from build123d import *

# Parameters (mm, degrees)
F0_W     = 64
F0_H     = 16
F1_DEPTH = 9
F2_R     = 2.5
F3_DEPTH = 2
F4_W     = 61
F4_H     = 13
F4_R     = 3.25
F4_R_2   = 2.5
F5_DEPTH = 8
F6_R     = 1.25
F7_DEPTH = 10


with BuildPart() as f1:
    # F0 (on Top) → F1 (new body)
    with BuildSketch(Plane.XY):
        Rectangle(F0_W, F0_H)
    extrude(amount=F1_DEPTH)

    # F2 (on face) → F3 (join)
    with BuildSketch(Plane.XY.offset(9)):
        with Locations((-28, 4)):
            Circle(F2_R)
        with Locations((-28, -4)):
            Circle(F2_R)
        with Locations((-20, 4)):
            Circle(F2_R)
        with Locations((-20, -4)):
            Circle(F2_R)
        with Locations((-12, 4)):
            Circle(F2_R)
        with Locations((-12, -4)):
            Circle(F2_R)
        with Locations((-4, 4)):
            Circle(F2_R)
        with Locations((-4, -4)):
            Circle(F2_R)
        with Locations((4, 4)):
            Circle(F2_R)
        with Locations((4, -4)):
            Circle(F2_R)
        with Locations((12, 4)):
            Circle(F2_R)
        with Locations((12, -4)):
            Circle(F2_R)
        with Locations((20, 4)):
            Circle(F2_R)
        with Locations((20, -4)):
            Circle(F2_R)
        with Locations((28, 4)):
            Circle(F2_R)
        with Locations((28, -4)):
            Circle(F2_R)
    extrude(amount=F3_DEPTH)

    # F4 (on face) → F5 (cut)
    with BuildSketch(Plane(origin=(0, 0, 0), x_dir=(1, 0, 0), z_dir=(0, 0, -1))):
        Rectangle(F4_W, F4_H)
        with Locations((-24, 0)):
            Circle(F4_R, mode=Mode.SUBTRACT)
        with Locations((-16, 0)):
            Circle(F4_R, mode=Mode.SUBTRACT)
        with Locations((-8, 0)):
            Circle(F4_R, mode=Mode.SUBTRACT)
        Circle(F4_R, mode=Mode.SUBTRACT)
        with Locations((8, 0)):
            Circle(F4_R, mode=Mode.SUBTRACT)
        with Locations((16, 0)):
            Circle(F4_R, mode=Mode.SUBTRACT)
        with Locations((24, 0)):
            Circle(F4_R, mode=Mode.SUBTRACT)
        with Locations((-24, 0)):
            Circle(F4_R_2)
        with Locations((-16, 0)):
            Circle(F4_R_2)
        with Locations((-8, 0)):
            Circle(F4_R_2)
        Circle(F4_R_2)
        with Locations((8, 0)):
            Circle(F4_R_2)
        with Locations((16, 0)):
            Circle(F4_R_2)
        with Locations((24, 0)):
            Circle(F4_R_2)
    extrude(amount=-F5_DEPTH, mode=Mode.SUBTRACT)

    # F6 (on face) → F7 (cut)
    with BuildSketch(Plane(origin=(0, 0, 0), x_dir=(1, 0, 0), z_dir=(0, 0, -1))):
        with Locations((-28, 4)):
            Circle(F6_R)
        with Locations((-28, -4)):
            Circle(F6_R)
        with Locations((-20, 4)):
            Circle(F6_R)
        with Locations((-20, -4)):
            Circle(F6_R)
        with Locations((-12, 4)):
            Circle(F6_R)
        with Locations((-12, -4)):
            Circle(F6_R)
        with Locations((-4, 4)):
            Circle(F6_R)
        with Locations((-4, -4)):
            Circle(F6_R)
        with Locations((4, 4)):
            Circle(F6_R)
        with Locations((4, -4)):
            Circle(F6_R)
        with Locations((12, 4)):
            Circle(F6_R)
        with Locations((12, -4)):
            Circle(F6_R)
        with Locations((20, 4)):
            Circle(F6_R)
        with Locations((20, -4)):
            Circle(F6_R)
        with Locations((28, 4)):
            Circle(F6_R)
        with Locations((28, -4)):
            Circle(F6_R)
    extrude(amount=-F7_DEPTH, mode=Mode.SUBTRACT)


solid = f1.part
Verification items for the finished model (mm, model axes). A direction names the side the tool comes from. Round coordinates to 2 decimals unless told otherwise and drop trailing zeros. Loops run counter-clockwise (first coordinate to the right, second up) from the corner with the lowest first, then second, coordinate; pieces in that order, holes last. Notation, with made-up numbers: (-33.75, 11) - (-6.75, 11) arc R31 ccw to (-6.75, 48) - close; hole circle Ø2 at (-16.5, 62). An arc over 180 degrees is marked (long way). Write item = value, one per line.
Q1. Sectioned sample at A-A on z = 4.5. State how many separate pieces and enclosed holes the cut face has, plus the area to 3 significant figures.
Here are the results:
separate_pieces = 8
enclosed_holes = 8
area = 326 mm^2
Q2. Tool access check on faces 1 (the cylindrical face through (4.577, 5.109, 8.986)), 2 (the flat face through (-12, 4, 11)), 3 (the cylindrical face through (-14.5, 4.1, 10)). Record the directions out of +Z, -Z, +X, -X, +Y, -Y that give a thin tool (end or side, any length) a straight path to the whole face; none if there is none.
Here are the results:
face_1 = -Z
face_2 = +Z, +X, -X, +Y, -Y
face_3 = +Z
Q3. Sectioned sample at B-B on x = -16. Record the boundary of the cut face in (y, z).
Here are the results:
outline = (-8, 0) - (-6.5, 0) - (-6.5, 8) - (-3.25, 8) - (-3.25, 0) - (-2.5, 0) - (-2.5, 8) - (2.5, 8) - (2.5, 0) - (3.25, 0) - (3.25, 8) - (6.5, 8) - (6.5, 0) - (8, 0) - (8, 9) - (-8, 9) - close
Q4. Depth check by flat-ended pin: pin 1 (2 mm diameter, centred on x = -28, y = 4, fed in from -Z); pin 2 (3 mm diameter, centred on x = 4, y = -4, fed in from -Z); pin 3 (6 mm diameter, centred on x = 24, y = 0, fed in from +Z). Enter the tip coordinate at first touch or a pass-through.
Here are the results:
pin_1 = 10
pin_2 = 8
pin_3 = 9
Q5. Material ranges on L1, parallel to Y at x = -12, z = 8.5; L2, parallel to Y at x = -16, z = 4; L3, parallel to Y at x = -20, z = 9.25, recorded low to high.
Here are the results:
L1 = -8 to -5.25, -2.75 to 2.75, 5.25 to 8
L2 = -8 to -6.5, -3.25 to -2.5, 2.5 to 3.25, 6.5 to 8
L3 = -6.5 to -5.25, -2.75 to -1.5, 1.5 to 2.75, 5.25 to 6.5
Q6. Sectioned sample at C-C on x = 20. Record the boundary of the cut face in (y, z), plus the area to 3 significant figures.
Here are the results:
outline = (-8, 0) - (-6.5, 0) - (-6.5, 8) - (-5.25, 8) - (-5.25, 10) - (-2.75, 10) - (-2.75, 8) - (2.75, 8) - (2.75, 10) - (5.25, 10) - (5.25, 8) - (6.5, 8) - (6.5, 0) - (8, 0) - (8, 9) - (6.5, 9) - (6.5, 11) - (1.5, 11) - (1.5, 9) - (-1.5, 9) - (-1.5, 11) - (-6.5, 11) - (-6.5, 9) - (-8, 9) - close
area = 50.0 mm^2
Q7. Mould release check, pull along X, two halves, no side actions. Record for faces 4 (the cylindrical face through (-26.845, 4.479, 8.986)), 5 (the flat face through (20, 4, 11)): +X half, -X half, draft (parallel to the pull), parting line (faces both ways), or undercut.
Here are the results:
face_4 = undercut
face_5 = draft
